from build123d import *

# Parameters (mm, degrees)
BOSS_EXTRUDE1_DEPTH = 31.75
SKETCH4_R           = 25.4
SKETCH4_R_2         = 23.8125
BOSS_EXTRUDE3_DEPTH = 12.7
SKETCH5_W           = 1.621707797
SKETCH5_H           = 1.5875
BOSS_EXTRUDE4_DEPTH = 25.4
SKETCH6_W           = 0.254
SKETCH6_H           = 0.254
BOSS_EXTRUDE5_DEPTH = 31.75
SKETCH9_R           = 25.4
SKETCH9_R_2         = 4.593847271
BOSS_EXTRUDE6_DEPTH = 6.35
SKETCH10_W          = 15.24
SKETCH10_H          = 41.544062962
SKETCH10_W_2        = 10.16
SKETCH10_H_2        = 36.95031579
BOSS_EXTRUDE7_DEPTH = 12.7
SKETCH11_W          = 15.24
SKETCH11_H          = 41.544062962
BOSS_EXTRUDE8_DEPTH = 2.54
FILLET1_R           = 2.54
FILLET2_R           = 2.54
CUT_EXTRUDE1_DEPTH  = 2.54


with BuildPart() as part:
    # Sketch2 → Boss-Extrude1 (new body)
    with BuildSketch(Plane.XY):
        with BuildLine():
            ThreePointArc((3.074180531, 0.79375), (-3.175, 0), (3.074180531, -0.79375))
            Line((3.074180531, -0.79375), (4.695888328, -0.79375))
            ThreePointArc((4.695888328, -0.79375), (-4.7625, 0), (4.695888328, 0.79375))
            Line((4.695888328, 0.79375), (3.074180531, 0.79375))
        make_face()
    extrude(amount=BOSS_EXTRUDE1_DEPTH)

    # Sketch5 → Boss-Extrude4 (add)
    with BuildSketch(Plane.XY):
        with Locations((3.88503443, 0)):
            Rectangle(SKETCH5_W, SKETCH5_H)
    extrude(amount=BOSS_EXTRUDE4_DEPTH)

    # Sketch6 → Boss-Extrude5 (add)
    with BuildSketch(Plane.XY):
        with BuildLine():
            Line((-1.306315103, 2.893815103), (-1.306315103, 1.306315103))
            Line((-1.306315103, 1.306315103), (-1.306315103, 1.052315103))
            Line((-1.306315103, 1.052315103), (-1.560315103, 1.052315103))
            Line((-1.560315103, 1.052315103), (-1.560315103, 1.306315103))
            Line((-1.560315103, 1.306315103), (-2.893815103, 1.306315103))
            ThreePointArc((-2.893815103, 1.306315103), (-2.428847118, 2.428847118), (-1.306315103, 2.893815103))
        make_face()
        with BuildLine():
            Line((1.306315103, 1.306315103), (2.893815103, 1.306315103))
            ThreePointArc((2.893815103, 1.306315103), (2.428847118, 2.428847118), (1.306315103, 2.893815103))
            Line((1.306315103, 2.893815103), (1.306315103, 1.306315103))
        make_face()
        with Locations((1.433315103, 1.179315103)):
            Rectangle(SKETCH6_W, SKETCH6_H)
    extrude(amount=BOSS_EXTRUDE5_DEPTH)



with BuildPart() as body_2:
    # Sketch4 → Boss-Extrude3 (new body)
    with BuildSketch(Plane.XY.offset(31.75)):
        Circle(SKETCH4_R)
        Circle(SKETCH4_R_2, mode=Mode.SUBTRACT)
    extrude(amount=-BOSS_EXTRUDE3_DEPTH)


with BuildPart() as part_1:
    add(part.part)

    add(body_2.part)  # Boss-Extrude6 merges body 2
    # Sketch9 → Boss-Extrude6 (add)
    with BuildSketch(Plane(origin=(0, 0, 19.05), x_dir=(-1, 0, 0), z_dir=(0, 0, -1))):
        with Locations(Location((0, 0, 0), (0, 0, 180))):
            Circle(SKETCH9_R)
        Circle(SKETCH9_R_2, mode=Mode.SUBTRACT)
    extrude(amount=BOSS_EXTRUDE6_DEPTH)

    # Sketch10 → Boss-Extrude7 (add)
    with BuildSketch(Plane(origin=(0, 0, 12.7), x_dir=(-1, 0, 0), z_dir=(0, 0, -1))):
        Rectangle(SKETCH10_W, SKETCH10_H)
        Rectangle(SKETCH10_W_2, SKETCH10_H_2, mode=Mode.SUBTRACT)
    extrude(amount=BOSS_EXTRUDE7_DEPTH)

    # Sketch11 → Boss-Extrude8 (add)
    with BuildSketch(Plane(origin=(0, 0, 0), x_dir=(-1, 0, 0), z_dir=(0, 0, -1))):
        Rectangle(SKETCH11_W, SKETCH11_H)
    extrude(amount=BOSS_EXTRUDE8_DEPTH)

    # Fillet1
    # the kernel refuses this fillet: 2.54 mm, written as the material it adds along each edge
    with BuildSketch(Plane(origin=(-7.62, -20.772031481, 12.7), x_dir=(-1, 0, 0), z_dir=(0, 1, 0)), Plane(origin=(7.62, 20.772031481, 12.7), x_dir=(1, 0, 0), z_dir=(0, -1, 0))) as fillet1_piece_1:
        with BuildLine():
            CenterArc((FILLET1_R, -FILLET1_R), FILLET1_R, 90, 90)
            Line((0, -FILLET1_R), (0, 0))
            Line((0, 0), (FILLET1_R, 0))
        make_face()
    extrude(amount=41.544062961)
    with BuildSketch(Plane(origin=(-7.62, 20.772031481, 12.7), x_dir=(0, 1, 0), z_dir=(1, 0, 0)), Plane(origin=(7.62, -20.772031481, 12.7), x_dir=(0, -1, 0), z_dir=(-1, 0, 0))) as fillet1_piece_2:
        with BuildLine():
            CenterArc((FILLET1_R, -FILLET1_R), FILLET1_R, 90, 90)
            Line((0, -FILLET1_R), (0, 0))
            Line((0, 0), (FILLET1_R, 0))
        make_face()
    extrude(amount=15.24)
    with BuildSketch(Plane(origin=(7.62, -20.772031481, 12.7), x_dir=(0, -1, 0), z_dir=(-1, 0, 0))) as fillet1_piece_3a_section:
        with BuildLine():
            CenterArc((FILLET1_R, -FILLET1_R), FILLET1_R, 90, 90)
            Line((0, -FILLET1_R), (0, 0))
            Line((0, 0), (FILLET1_R, 0))
        make_face()
    fillet1_piece_3a = extrude(amount=21.59, mode=Mode.PRIVATE)
    fillet1_piece_3a = fillet1_piece_3a & Plane(origin=(0, 0, 12.091015905), x_dir=(1, 0, 0), z_dir=(0, 0, 1)) * Cylinder(25.4, 54, mode=Mode.PRIVATE)
    fillet1_piece_3a = split(fillet1_piece_3a, bisect_by=Plane(origin=(-7.62, -21.280779279, 12.091015905), z_dir=(-1, 0, 0)), keep=Keep.TOP, mode=Mode.PRIVATE)
    with BuildSketch(Plane(origin=(-7.62, -27.122031481, 12.7), x_dir=(-1, 0, 0), z_dir=(0, 1, 0))) as fillet1_piece_3b_section:
        with BuildLine():
            CenterArc((FILLET1_R, -FILLET1_R), FILLET1_R, 90, 90)
            Line((0, -FILLET1_R), (0, 0))
            Line((0, 0), (FILLET1_R, 0))
        make_face()
    fillet1_piece_3b = extrude(amount=47.894062961, mode=Mode.PRIVATE)
    fillet1_piece_3b = fillet1_piece_3b & Plane(origin=(0, 0, 12.105999198), x_dir=(1, 0, 0), z_dir=(0, 0, 1)) * Cylinder(25.4, 106, mode=Mode.PRIVATE)
    fillet1_piece_3b = split(fillet1_piece_3b, bisect_by=Plane(origin=(-8.162359675, -20.772031481, 12.105999198), z_dir=(0, -1, 0)), keep=Keep.TOP, mode=Mode.PRIVATE)
    fillet1_piece_3 = fillet1_piece_3a & fillet1_piece_3b
    add(fillet1_piece_3)
    with BuildSketch(Plane(origin=(-7.62, -20.772031481, 12.7), x_dir=(-1, 0, 0), z_dir=(0, 1, 0))) as fillet1_piece_4a_section:
        with BuildLine():
            CenterArc((FILLET1_R, -FILLET1_R), FILLET1_R, 90, 90)
            Line((0, -FILLET1_R), (0, 0))
            Line((0, 0), (FILLET1_R, 0))
        make_face()
    fillet1_piece_4a = extrude(amount=47.894062961, mode=Mode.PRIVATE)
    fillet1_piece_4a = fillet1_piece_4a & Plane(origin=(0, 0, 12.105997934), x_dir=(1, 0, 0), z_dir=(0, 0, 1)) * Cylinder(25.4, 106, mode=Mode.PRIVATE)
    fillet1_piece_4a = split(fillet1_piece_4a, bisect_by=Plane(origin=(-8.162364443, 20.772031481, 12.105997934), z_dir=(0, 1, 0)), keep=Keep.TOP, mode=Mode.PRIVATE)
    with BuildSketch(Plane(origin=(-13.97, 20.772031481, 12.7), x_dir=(0, 1, 0), z_dir=(1, 0, 0))) as fillet1_piece_4b_section:
        with BuildLine():
            CenterArc((FILLET1_R, -FILLET1_R), FILLET1_R, 90, 90)
            Line((0, -FILLET1_R), (0, 0))
            Line((0, 0), (FILLET1_R, 0))
        make_face()
    fillet1_piece_4b = extrude(amount=21.59, mode=Mode.PRIVATE)
    fillet1_piece_4b = fillet1_piece_4b & Plane(origin=(0, 0, 12.0910159), x_dir=(1, 0, 0), z_dir=(0, 0, 1)) * Cylinder(25.4, 54, mode=Mode.PRIVATE)
    fillet1_piece_4b = split(fillet1_piece_4b, bisect_by=Plane(origin=(-7.62, 21.28077831, 12.0910159), z_dir=(-1, 0, 0)), keep=Keep.TOP, mode=Mode.PRIVATE)
    fillet1_piece_4 = fillet1_piece_4a & fillet1_piece_4b
    add(fillet1_piece_4)
    with BuildSketch(Plane(origin=(-7.62, 20.772031481, 12.7), x_dir=(0, 1, 0), z_dir=(1, 0, 0))) as fillet1_piece_5a_section:
        with BuildLine():
            CenterArc((FILLET1_R, -FILLET1_R), FILLET1_R, 90, 90)
            Line((0, -FILLET1_R), (0, 0))
            Line((0, 0), (FILLET1_R, 0))
        make_face()
    fillet1_piece_5a = extrude(amount=21.59, mode=Mode.PRIVATE)
    fillet1_piece_5a = fillet1_piece_5a & Plane(origin=(0, 0, 12.091015905), x_dir=(1, 0, 0), z_dir=(0, 0, 1)) * Cylinder(25.4, 54, mode=Mode.PRIVATE)
    fillet1_piece_5a = split(fillet1_piece_5a, bisect_by=Plane(origin=(7.62, 21.280779279, 12.091015905), z_dir=(1, 0, 0)), keep=Keep.TOP, mode=Mode.PRIVATE)
    with BuildSketch(Plane(origin=(7.62, 27.122031481, 12.7), x_dir=(1, 0, 0), z_dir=(0, -1, 0))) as fillet1_piece_5b_section:
        with BuildLine():
            CenterArc((FILLET1_R, -FILLET1_R), FILLET1_R, 90, 90)
            Line((0, -FILLET1_R), (0, 0))
            Line((0, 0), (FILLET1_R, 0))
        make_face()
    fillet1_piece_5b = extrude(amount=47.894062961, mode=Mode.PRIVATE)
    fillet1_piece_5b = fillet1_piece_5b & Plane(origin=(0, 0, 12.105999198), x_dir=(1, 0, 0), z_dir=(0, 0, 1)) * Cylinder(25.4, 106, mode=Mode.PRIVATE)
    fillet1_piece_5b = split(fillet1_piece_5b, bisect_by=Plane(origin=(8.162359675, 20.772031481, 12.105999198), z_dir=(0, 1, 0)), keep=Keep.TOP, mode=Mode.PRIVATE)
    fillet1_piece_5 = fillet1_piece_5a & fillet1_piece_5b
    add(fillet1_piece_5)
    with BuildSketch(Plane(origin=(13.97, -20.772031481, 12.7), x_dir=(0, -1, 0), z_dir=(-1, 0, 0))) as fillet1_piece_6a_section:
        with BuildLine():
            CenterArc((FILLET1_R, -FILLET1_R), FILLET1_R, 90, 90)
            Line((0, -FILLET1_R), (0, 0))
            Line((0, 0), (FILLET1_R, 0))
        make_face()
    fillet1_piece_6a = extrude(amount=21.59, mode=Mode.PRIVATE)
    fillet1_piece_6a = fillet1_piece_6a & Plane(origin=(0, 0, 12.0910159), x_dir=(1, 0, 0), z_dir=(0, 0, 1)) * Cylinder(25.4, 54, mode=Mode.PRIVATE)
    fillet1_piece_6a = split(fillet1_piece_6a, bisect_by=Plane(origin=(7.62, -21.28077831, 12.0910159), z_dir=(1, 0, 0)), keep=Keep.TOP, mode=Mode.PRIVATE)
    with BuildSketch(Plane(origin=(7.62, 20.772031481, 12.7), x_dir=(1, 0, 0), z_dir=(0, -1, 0))) as fillet1_piece_6b_section:
        with BuildLine():
            CenterArc((FILLET1_R, -FILLET1_R), FILLET1_R, 90, 90)
            Line((0, -FILLET1_R), (0, 0))
            Line((0, 0), (FILLET1_R, 0))
        make_face()
    fillet1_piece_6b = extrude(amount=47.894062961, mode=Mode.PRIVATE)
    fillet1_piece_6b = fillet1_piece_6b & Plane(origin=(0, 0, 12.105997934), x_dir=(1, 0, 0), z_dir=(0, 0, 1)) * Cylinder(25.4, 106, mode=Mode.PRIVATE)
    fillet1_piece_6b = split(fillet1_piece_6b, bisect_by=Plane(origin=(8.162364443, -20.772031481, 12.105997934), z_dir=(0, -1, 0)), keep=Keep.TOP, mode=Mode.PRIVATE)
    fillet1_piece_6 = fillet1_piece_6a & fillet1_piece_6b
    add(fillet1_piece_6)

    # Fillet2
    fillet2_edges = [part_1.edges().sort_by_distance(p)[0] for p in [
        (-7.62, 0, -2.54),
        (0, 20.772031481, -2.54),
        (7.62, 0, -2.54),
        (0, -20.772031481, -2.54),
    ]]
    fillet(fillet2_edges, radius=FILLET2_R)

    # Sketch12 → Cut-Extrude1 (cut)
    with BuildSketch(Plane(origin=(0, 0, 12.7), x_dir=(-1, 0, 0), z_dir=(0, 0, -1))):
        with BuildLine():
            Line((16.813868884, 14.704492606), (17.547564981, 16.722156872))
            Line((17.547564981, 16.722156872), (18.489141639, 14.704492606))
            add(Edge.make_bspline(
                [(18.489141639, 14.704492606), (19.798776644, 12.786117496), (18.310846307, 9.647278033), (13.185757244, 9.226397866), (12.693603367, 13.337843102), (13.512236449, 14.704492606)],
                knots=[0, 0, 0, 0, 0.432949875, 0.596956743, 1, 1, 1, 1], degree=3))
            Line((13.512236449, 14.704492606), (14.00136718, 16.691586201))
            Line((14.00136718, 16.691586201), (14.612780594, 14.704492606))
            Line((14.612780594, 14.704492606), (15.591042056, 18.678679797))
            Line((15.591042056, 18.678679797), (16.813868884, 14.704492606))
        make_face()
        Polygon((22.65270588, 5.371871988), (23.452991012, 5.371871988), (23.452991012, -1.999175277), (22.65270588, -1.999175277), (22.65270588, 1.033484169), (20.757293726, 1.033484169), (20.757293726, -1.999175277), (19.662166704, -1.999175277), (19.662166704, 5.371871988), (20.757293726, 5.371871988), (20.757293726, 2.549813892), (22.65270588, 2.549813892), align=None)
        Polygon((-23.636155952, 5.371871988), (-23.636155952, -1.999175277), (-19.528236773, -1.999175277), (-19.528236773, -0.945591056), (-22.125891548, -0.945591056), (-22.125891548, 5.371871988), align=None)
    extrude(amount=-CUT_EXTRUDE1_DEPTH, mode=Mode.SUBTRACT)


solid = part_1.part
Design review of the part built by this model. Coordinates are the model's own, in mm. A direction names the side the tool comes from. Coordinates: 2 decimals unless noted, no trailing zeros. Loops run counter-clockwise (first coordinate to the right, second up) from the corner with the lowest first, then second, coordinate; pieces in that order, holes last.
Item 1: For faces 1 (the cylindrical face through (-6.896, 0.291, -1.776)), 2 (the flat face through (4.696, 0, 6)), 3 (the flat face through (0, 24, 12.7)), 4 (the flat face through (3.074, 0, 13)), 5 (the flat face through (-23, -7, 31.75)), list the 3-axis set-ups (+Z, -Z, +X, -X, +Y, -Y) from which the entire face can be reached by the end or side of a thin tool; tool diameter is ignored.
Completed:
face 1: -Z, -X, +Y, -Y
face 2: none
face 3: -Z, +X, -X, +Y
face 4: +Z
face 5: +Z, +X, -X, +Y, -Y
Item 2: Draft analysis for pull direction Y (two halves, no side actions). For faces 6 (the flat face through (1.306, 2, 16)), 7 (the flat face through (-22, 2.55, 14)), 8 (the flat face through (0, 20.772, 5)), 9 (the flat face through (0, -20.772, 5)), state which applies: pulls with the +Y half, pulls with the -Y half, needs draft (parallel to the pull), parting line crosses it, or undercut.
Completed:
face 6: undercut
face 7: undercut
face 8: pulls with the +Y half
face 9: pulls with the -Y half
Item 3: Add section C-C (y = -7). Write out the cut boundary in (x, z), and give its area (3 significant figures).
Completed:
outline: (-24.42, 12.7) - (-10.16, 12.7) arc R2.54 cw to (-7.62, 10.16) - (-7.62, 0) arc R2.54 ccw to (-5.08, -2.54) - (5.08, -2.54) arc R2.54 ccw to (7.62, 0) - (7.62, 10.16) arc R2.54 cw to (10.16, 12.7) - (24.42, 12.7) - (24.42, 31.75) - (22.76, 31.75) - (22.76, 19.05) - (-22.76, 19.05) - (-22.76, 31.75) - (-24.42, 31.75) - close; hole (-5.08, 0) - (5.08, 0) - (5.08, 12.7) - (-5.08, 12.7) - close
area: 455 mm2
Item 4: Clearance check with flat-ended pins moving along their axes: pin 1 (8 mm diameter, centred on x = -1.5, z = 5.5, fed in from -Y); pin 2 (2 mm diameter, centred on y = -4, z = 3.5, fed in from -X); pin 3 (2 mm diameter, centred on x = -18, z = 17, fed in from +Y). State where each tip first meets the part, or that it passes through.
Completed:
pin 1: stops at y = -20.77
pin 2: stops at x = -7.62
pin 3: stops at y = 18.87
Item 5: Add section A-A (z = 7). Give the number of separate pieces and of enclosed holes in the cut face, and give its area (3 significant figures).
Completed:
separate pieces: 2
enclosed holes: 2
area: 301 mm2
Item 6: Wall thickness on L1, parallel to Y at x = 0, z = 25 (1 decimal); L2, parallel to Y at x = 0, z = 8 (1 decimal); L3, parallel to X at y = 2, z = 1: over which ranges is each line inside the solid? List them lowest first.
Completed:
L1: y = -25.4 to -23.8, -4.8 to -3.2, 3.2 to 4.8, 23.8 to 25.4
L2: y = -20.8 to -18.5, -4.8 to -3.2, 3.2 to 4.8, 18.5 to 20.8
L3: x = -7.62 to -5.08, -4.32 to -1.31, 1.31 to 4.32, 5.08 to 7.62
